Here's how the part is built. I have some questions about the finished solid (model axes, mm). Face numbers are marked on the shaded views. A direction names the side the tool comes from. Round coordinates to 2 decimals unless told otherwise and drop trailing zeros. Loops run counter-clockwise (first coordinate to the right, second up) from the corner with the lowest first, then second, coordinate; pieces in that order, holes last. Notation, with made-up numbers: M 46,70 L 104,70 A19 cw 104,85 Z; hole C 87.5,-14 d9. An arc over 180 degrees is marked long. Write each question's results on one line, items separated by ' | '. Start each with the question number.
```python
from build123d import *

# Parameters (mm, degrees)
BOSS_EXTRUDE1_DEPTH = 2


with BuildPart() as part:
    # Sketch1 → Boss-Extrude1 (new body)
    with BuildSketch(Plane(origin=(0, 0, 0), x_dir=(1, 0, 0), z_dir=(0, 1, 0))):
        Polygon((0, 0), (20.112843107, 5.220264813), (29.03786322, 5.220264813), (29.03786322, 7.220264813), (29.03786322, 7.536743304), (28.284188889, 10.440529626), (15.877025026, 7.220264813), (-0.75367433, 7.220264813), (-0.75367433, 5.220264813), (-0.75367433, 2.903786322), align=None)
        with BuildLine():
            Line((0.516929559, 4.720264813), (0.516929559, 4.186250024))
            ThreePointArc((0.516929559, 4.186250024), (0.71099345, 3.79077171), (1.142541948, 3.702285637))
            Line((1.142541948, 3.702285637), (3.200015285, 4.236300426))
            ThreePointArc((3.200015285, 4.236300426), (3.570377792, 4.783580714), (3.074402897, 5.220264813))
            Line((3.074402897, 5.220264813), (1.016929559, 5.220264813))
            ThreePointArc((1.016929559, 5.220264813), (0.663376169, 5.073818204), (0.516929559, 4.720264813))
        make_face(mode=Mode.SUBTRACT)
    extrude(amount=BOSS_EXTRUDE1_DEPTH)


solid = part.part
```
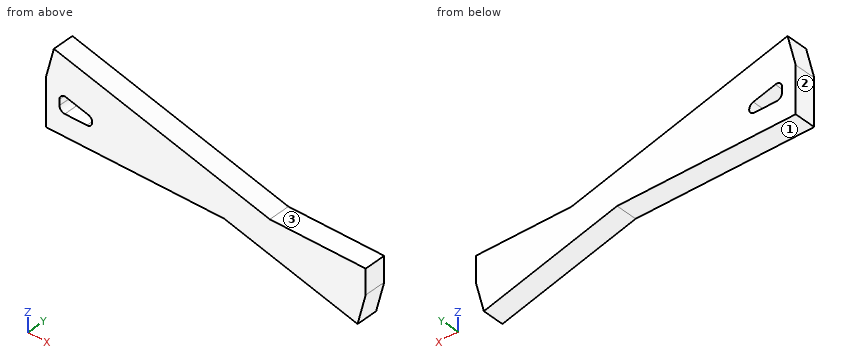
Item 1: I'm going to push flat-ended pins straight in: pin 1 (1.5 mm diameter, centred on x = 8.5, z = -2.5, fed in from -Y); pin 2 (1 mm diameter, centred on x = 9, y = 1, fed in from -Z). Where does each tip first touch, or does it pass through?
Item 2: If we section it at A-A on y = 1.6: Please give me the cut outline in (x, z), and give its area (3 significant figures).
Item 3: If we section it at D-D on x = 8.25: Please give me the cut outline in (y, z).
Item 4: I need wall thicknesses on L1, parallel to Z at x = 2.75, y = 0.2; L2, parallel to Z at x = 3.75, y = 0.3; L3, parallel to Z at x = 19, y = 1.7. Which ranges of each line are inside material? Lowest first, please.
Item 5: If we section it at C-C on z = -2.5: Please give me the cut outline in (x, y).
Item 6: Which directions (+Z, -Z, +X, -X, +Y, -Y) give clear straight access to the entire face, cutting with the end or side of a thin tool? Please do the marked faces 1, 2 and 3.
Item 7: If we section it at B-B on x = 2: Please give me the cut outline in (y, z).
Numbers:
1) pin 1: y = 0 | pin 2: z = -7.22
2) outline: M -0.75,-7.22 L 15.88,-7.22 L 28.28,-10.44 L 29.04,-7.54 L 29.04,-5.22 L 20.11,-5.22 L 0,0 L -0.75,-2.9 Z; hole M 0.52,-4.72 A0.5 ccw 1.02,-5.22 L 3.07,-5.22 A0.5 ccw 3.2,-4.24 L 1.14,-3.7 A0.5 ccw 0.52,-4.19 Z | area: 133 mm²
3) outline: M 0,-7.22 L 2,-7.22 L 2,-2.14 L 0,-2.14 Z
4) L1: -7.22 to -5.22, -4.12 to -0.71 | L2: -7.22 to -0.97 | L3: -8.03 to -4.93
5) outline: M -0.65,0 L 9.63,0 L 9.63,2 L -0.65,2 Z
6) face 1: -Z, -X, +Y, -Y | face 2: +Z, -Z, -X, +Y, -Y | face 3: +Z, +X, +Y, -Y
7) outline: M 0,-7.22 L 2,-7.22 L 2,-5.22 L 0,-5.22 Z; M 0,-3.92 L 2,-3.92 L 2,-0.52 L 0,-0.52 Z
